Source: CAD feature listing. Evaluate the final solid. Frame: model axes, mm. Give positions to 0.01 mm unless a question says otherwise; leave off trailing zeros. Loops run counter-clockwise (first coordinate to the right, second up) from the corner with the lowest first, then second, coordinate; pieces in that order, holes last. Notation, with made-up numbers: (14.25, -37.5) -> (53.25, -37.5) arc R22 ccw to (53.25, -16.5) -> close; hole circle Ø11 at (-12.75, -28). An arc over 180 degrees is marked (long way). Put each result on its own line as item: value.
```python
from build123d import *

# Parameters (mm, degrees)
PARED_A_MOTOR_J2_START           = 67.85
CROQUIS1_W                       = 90
CROQUIS1_H                       = 81.25
PARED_A_MOTOR_J2_DEPTH           = 6.35
PARED_A_MOTOR_J2_REDONDEO_START  = 67.85
CROQUIS2_R                       = 45
PARED_A_MOTOR_J2_REDONDEO_DEPTH  = 6.35
ROSCA_M3_ESCUADRAS_START         = 67.85
CROQUIS4_R                       = 1.25
ROSCA_M3_ESCUADRAS_DEPTH         = 6.35
PASADORES_D4_START               = 90.2
CROQUIS5_R                       = 2
PASADORES_D4_DEPTH               = 8
ROSCA_M3_BASES_CINCHO_START      = 67.85
CROQUIS6_R                       = 1.25
ROSCA_M3_BASES_CINCHO_DEPTH      = 6.35
PASO_DRIVER_Y_8XM3_START         = 67.85
CROQUIS7_R                       = 30
CROQUIS7_R_2                     = 1.7
PASO_DRIVER_Y_8XM3_DEPTH         = 6.35
PASO_M3_ESCUADRAS_TUERCA_START   = 67.85
CROQUIS8_R                       = 1.7
PASO_M3_ESCUADRAS_TUERCA_DEPTH   = 6.35
PASO_M3_BASE_CINCHO_TUERCA_START = 67.85
CROQUIS9_R                       = 1.7
PASO_M3_BASE_CINCHO_TUERCA_DEPTH = 6.35


with BuildPart() as part:
    # Croquis1 → Pared_A_motor_J2 (new body)
    with BuildSketch(Plane(origin=(0, 0, 0), x_dir=(1, 0, 0), z_dir=(0, 1, 0)).offset(PARED_A_MOTOR_J2_START)):
        with Locations((0, -130.825)):
            Rectangle(CROQUIS1_W, CROQUIS1_H)
    extrude(amount=PARED_A_MOTOR_J2_DEPTH)

    # Croquis2 → Pared_A_motor_J2_redondeo (add)
    with BuildSketch(Plane(origin=(0, 0, 0), x_dir=(1, 0, 0), z_dir=(0, 1, 0)).offset(PARED_A_MOTOR_J2_REDONDEO_START)):
        with Locations((0, -171.45)):
            Circle(CROQUIS2_R)
    extrude(amount=PARED_A_MOTOR_J2_REDONDEO_DEPTH)

    # Croquis4 → Rosca_M3_escuadras (cut)
    with BuildSketch(Plane(origin=(0, 0, 0), x_dir=(1, 0, 0), z_dir=(0, 1, 0)).offset(ROSCA_M3_ESCUADRAS_START)):
        with Locations(Location((-25, -105.2, 0), (0, 0, 90))):
            Circle(CROQUIS4_R)
        with Locations(Location((25, -105.2, 0), (0, 0, 90))):
            Circle(CROQUIS4_R)
    extrude(amount=ROSCA_M3_ESCUADRAS_DEPTH, mode=Mode.SUBTRACT)

    # Croquis5 → Pasadores_D4 (cut)
    with BuildSketch(Plane.XY.offset(PASADORES_D4_START)):
        with Locations((-38, 71.025)):
            Circle(CROQUIS5_R)
        with Locations((38, 71.025)):
            Circle(CROQUIS5_R)
    extrude(amount=PASADORES_D4_DEPTH, mode=Mode.SUBTRACT)

    # Croquis6 → Rosca_M3_bases_cincho (cut)
    with BuildSketch(Plane(origin=(0, 0, 0), x_dir=(1, 0, 0), z_dir=(0, 1, 0)).offset(ROSCA_M3_BASES_CINCHO_START)):
        with Locations(Location((0, -117, 0), (0, 0, 90))):
            Circle(CROQUIS6_R)
    extrude(amount=ROSCA_M3_BASES_CINCHO_DEPTH, mode=Mode.SUBTRACT)

    # Croquis7 → Paso_driver_y_8xM3 (cut)
    with BuildSketch(Plane(origin=(0, 0, 0), x_dir=(1, 0, 0), z_dir=(0, 1, 0)).offset(PASO_DRIVER_Y_8XM3_START)):
        with Locations(Location((0, -171.45, 0), (0, 0, 90))):
            Circle(CROQUIS7_R)
        with Locations(Location((34.401729978, -185.070608449, 0), (0, 0, 90))):
            Circle(CROQUIS7_R_2)
        with Locations(Location((14.694471953, -205.40692115, 0), (0, 0, 90))):
            Circle(CROQUIS7_R_2)
        with Locations(Location((-13.620608449, -205.851729978, 0), (0, 0, 90))):
            Circle(CROQUIS7_R_2)
        with Locations(Location((-33.95692115, -186.144471953, 0), (0, 0, 90))):
            Circle(CROQUIS7_R_2)
        with Locations(Location((-34.401729978, -157.829391551, 0), (0, 0, 90))):
            Circle(CROQUIS7_R_2)
        with Locations(Location((-14.694471953, -137.49307885, 0), (0, 0, 90))):
            Circle(CROQUIS7_R_2)
        with Locations(Location((13.620608449, -137.048270022, 0), (0, 0, 90))):
            Circle(CROQUIS7_R_2)
        with Locations(Location((33.95692115, -156.755528047, 0), (0, 0, 90))):
            Circle(CROQUIS7_R_2)
    extrude(amount=PASO_DRIVER_Y_8XM3_DEPTH, mode=Mode.SUBTRACT)

    # Croquis8 → Paso_M3_escuadras_tuerca (cut)
    with BuildSketch(Plane(origin=(0, 0, 0), x_dir=(1, 0, 0), z_dir=(0, 1, 0)).offset(PASO_M3_ESCUADRAS_TUERCA_START)):
        with Locations(Location((-25, -105.2, 0), (0, 0, 90))):
            Circle(CROQUIS8_R)
        with Locations(Location((25, -105.2, 0), (0, 0, 90))):
            Circle(CROQUIS8_R)
    extrude(amount=PASO_M3_ESCUADRAS_TUERCA_DEPTH, mode=Mode.SUBTRACT)

    # Croquis9 → Paso_M3_base_cincho_tuerca (cut)
    with BuildSketch(Plane(origin=(0, 0, 0), x_dir=(1, 0, 0), z_dir=(0, 1, 0)).offset(PASO_M3_BASE_CINCHO_TUERCA_START)):
        with Locations(Location((0, -117, 0), (0, 0, 90))):
            Circle(CROQUIS9_R)
    extrude(amount=PASO_M3_BASE_CINCHO_TUERCA_DEPTH, mode=Mode.SUBTRACT)


solid = part.part
```
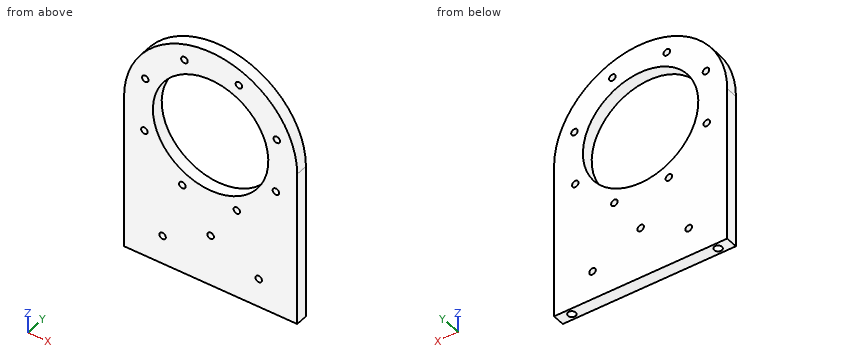
(1) Section C-C on y = 72. Give the number of separate pieces and of enclosed holes in the cut face, then the cut area to 3 significant figures.
Calculated:
separate pieces: 1
enclosed holes: 12
area: 7,510 mm²
(2) Section A-A on x = 0. Return loops of the section in (y, z), then the cut area to 3 significant figures.
Calculated:
outline: (67.85, 90.2) -> (74.2, 90.2) -> (74.2, 115.3) -> (67.85, 115.3) -> close; (67.85, 118.7) -> (74.2, 118.7) -> (74.2, 141.45) -> (67.85, 141.45) -> close; (67.85, 201.45) -> (74.2, 201.45) -> (74.2, 216.45) -> (67.85, 216.45) -> close
area: 399 mm²
(3) Section B-B on z = 117. Return loops of the section in (x, y), then the cut area to 3 significant figures.
Calculated:
outline: (-45, 67.85) -> (-1.7, 67.85) -> (-1.7, 74.2) -> (-45, 74.2) -> close; (1.7, 67.85) -> (45, 67.85) -> (45, 74.2) -> (1.7, 74.2) -> close
area: 550 mm²
(4) Section D-D on z = 137.5. Return loops of the section in (x, y), then the cut area to 3 significant figures.
Calculated:
outline: (-45, 67.85) -> (-16.39, 67.85) -> (-16.39, 74.2) -> (-45, 74.2) -> close; (-12.99, 67.85) -> (11.98, 67.85) -> (11.98, 74.2) -> (-12.99, 74.2) -> close; (15.26, 67.85) -> (45, 67.85) -> (45, 74.2) -> (15.26, 74.2) -> close
area: 529 mm²
(5) Line query: probe 1 along X at (y, z) = (71.25, 105.2); probe 2 along Z at (x, y) = (-16, 68.75); probe 3 along X at (y, z) = (72, 171.45). Output: solid intervals per line, ascending. Write a range as from..to.
Calculated:
probe 1: x = -45..-26.7, -23.3..23.3, 26.7..45
probe 2: z = 90.2..136.4, 138.58..146.07, 196.83..213.51
probe 3: x = -45..-30, 30..45
